from build123d import *

# Parameters (mm, degrees)
SKETCH1_W          = 9.525
SKETCH1_H          = 2.0828
CHAMFER1_SIZE      = 0.5953125
CUT_EXTRUDE2_DEPTH = 1.99136


with BuildPart() as part:
    # Sketch1 → Revolve1 (revolve)
    with BuildSketch(Plane(origin=(0, 0, 0), x_dir=(0, 0, -1), z_dir=(1, 0, 0))):
        with Locations((4.7625, 1.0414)):
            Rectangle(SKETCH1_W, SKETCH1_H)
    revolve(axis=Axis((0, 0, -9.525), (0, 0, 1)))

    # Chamfer1
    chamfer1_edges = [part.edges().sort_by_distance(p)[0] for p in [
        (0, -2.0828, -9.525),
    ]]
    chamfer(chamfer1_edges, length=CHAMFER1_SIZE)

    # Sketch7 → Revolve2 (revolve)
    with BuildSketch(Plane(origin=(0, 0, 0), x_dir=(0, 0, -1), z_dir=(1, 0, 0)), mode=Mode.PRIVATE) as revolve2_sk:
        with BuildLine():
            Line((0, 4.5593), (0.28448, 4.5593))
            Line((0.28448, 4.5593), (2.8448, 2.333647779))
            ThreePointArc((2.8448, 2.333647779), (3.157581097, 2.147562581), (3.515722863, 2.0828))
            Line((3.515722863, 2.0828), (3.515722863, 0))
            Line((3.515722863, 0), (0, 0))
            Line((0, 0), (0, 4.5593))
        make_face()
    revolve(revolve2_sk.sketch.rotate(Axis((0, 0, 0), (0, 0, -1)), 180), axis=Axis((0, 0, 0), (0, 0, -1)))

    # Boss-Extrude1 cone 1 section (through the dimple's axis) → Boss-Extrude1 (revolve)
    with BuildSketch(Plane(origin=(0, 0, -3.515722863), x_dir=(0, -1, 0), z_dir=(1, 0, 0))):
        Polygon((0, 0), (2.0828, 0), (0, 2.0828), align=None)
    revolve(axis=Axis((0, 0, -3.515722863), (0, 0, -1)))

    # Sketch5 → Cut-Extrude2 (cut)
    with BuildSketch(Plane.XY):
        Polygon((1.190625, -0.687407664), (1.190625, 0.687407664), (0, 1.374815329), (-1.190625, 0.687407664), (-1.190625, -0.687407664), (0, -1.374815329), align=None)
    extrude(amount=-CUT_EXTRUDE2_DEPTH, mode=Mode.SUBTRACT)

    # Cut-Extrude3 cone 1 section (through the dimple's axis) → Cut-Extrude3 (revolve, cut)
    with BuildSketch(Plane(origin=(0, 0, 0), x_dir=(0, -1, 0), z_dir=(1, 0, 0))):
        Polygon((0, 0), (1.374815329, 0), (0, 1.374815329), align=None)
    revolve(axis=Axis((0, 0, 0), (0, 0, -1)), mode=Mode.SUBTRACT)


solid = part.part
Part model, mm, in its own coordinate system. A direction names the side the tool comes from. Coordinates: 2 decimals unless noted, no trailing zeros. Loops run counter-clockwise (first coordinate to the right, second up) from the corner with the lowest first, then second, coordinate; pieces in that order, holes last. Notation, with made-up numbers: (20.5, 85) -> (24.5, 85) arc R12 cw to (24.5, 102) -> close; hole circle Ø4 at (5.5, -34). An arc over 180 degrees is marked (long way). Use a Markdown table: item, result. Add a question column.
Item 1: Band-saw the part on C-C on z = -8.5. Write the cut outline in (x, y).
Item 2: Flat gauge pins, fed straight in: P1, Ø1, axis at x = -2.5, z = -2, coming from the -Y side; P2, Ø4, axis at x = -2.5, z = -6.5, coming from the +Y side; P3, Ø4, axis at x = 2, z = -4.5, coming from the +Y side; P4, Ø2, axis at x = 3, y = 2.5, coming from the +Z side. Where does each tip first touch, or does it go through?
Item 3: Probe probe 1 along X at (y, z) = (-1.25, -0.5); probe 2 along X at (y, z) = (-1.25, -1.75); probe 3 along X at (y, z) = (2, -1.25). List the from-to ranges inside material, lowest first.
Item 4: Which spindle directions (+Z, -Z, +X, -X, +Y, -Y) get a long thin tool onto all of the face, cutting with end or side? Do faces 1 (the cylindrical face through (-0.626, 1.987, -6.261)), 2 (the flat face through (0.587, -1.036, -0.982)), 3 (the flat face through (0, 0, -9.525)). Say none if no direction does.
Item 5: Band-saw the part on B-B on z = -1. Write the cut outline in (x, y).
Item 6: Pull direction Y, two halves, no side cores. Call faces 4 (the conical face through (-0.73, -2.33, -2.72)), 5 (the flat face through (0.6, 1.03, -0.98)), 6 (the flat face through (1.191, 0, -1)), 7 (the flat face through (-1.1, -1.1, 0)): +Y half, -Y half, draft (parallel to the pull), parting line (faces both ways), or undercut.
Item 7: Band-saw the part on A-A on y = 0. Write the cut outline in (x, z) (3 decimals).
Geometry says:
| question | item | result |
|---|---|---|
| 1 | outline | circle Ø4.17 at (0, 0) |
| 2 | P1 | y = -2.61 |
| 2 | P2 | y = 2.02 |
| 2 | P3 | y = 2.19 |
| 2 | P4 | z = 0 |
| 3 | probe 1 | -4.19 to -0.22, 0.22 to 4.19 |
| 3 | probe 2 | -3.04 to -0.22, 0.22 to 3.04 |
| 3 | probe 3 | -3.14 to 3.14 |
| 4 | face 1 | -Z |
| 4 | face 2 | +Z |
| 4 | face 3 | -Z, +X, -X, +Y, -Y |
| 5 | outline | circle Ø7.87 at (0, 0); hole (-1.19, -0.69) -> (0, -1.37) -> (1.19, -0.69) -> (1.19, 0.69) -> (0, 1.37) -> (-1.19, 0.69) -> close |
| 6 | face 4 | parting line |
| 6 | face 5 | undercut |
| 6 | face 6 | undercut |
| 6 | face 7 | draft |
| 7 | outline | (-4.559, -0.284) -> (-2.334, -2.845) arc R1.023 cw to (-2.083, -3.516) -> (-2.083, -8.93) -> (-1.487, -9.525) -> (1.487, -9.525) -> (2.083, -8.93) -> (2.083, -3.516) arc R1.023 cw to (2.334, -2.845) -> (4.559, -0.284) -> (4.559, 0) -> (1.375, 0) -> (1.191, -0.184) -> (1.191, -1.991) -> (-1.191, -1.991) -> (-1.191, -0.184) -> (-1.375, 0) -> (-4.559, 0) -> close |
